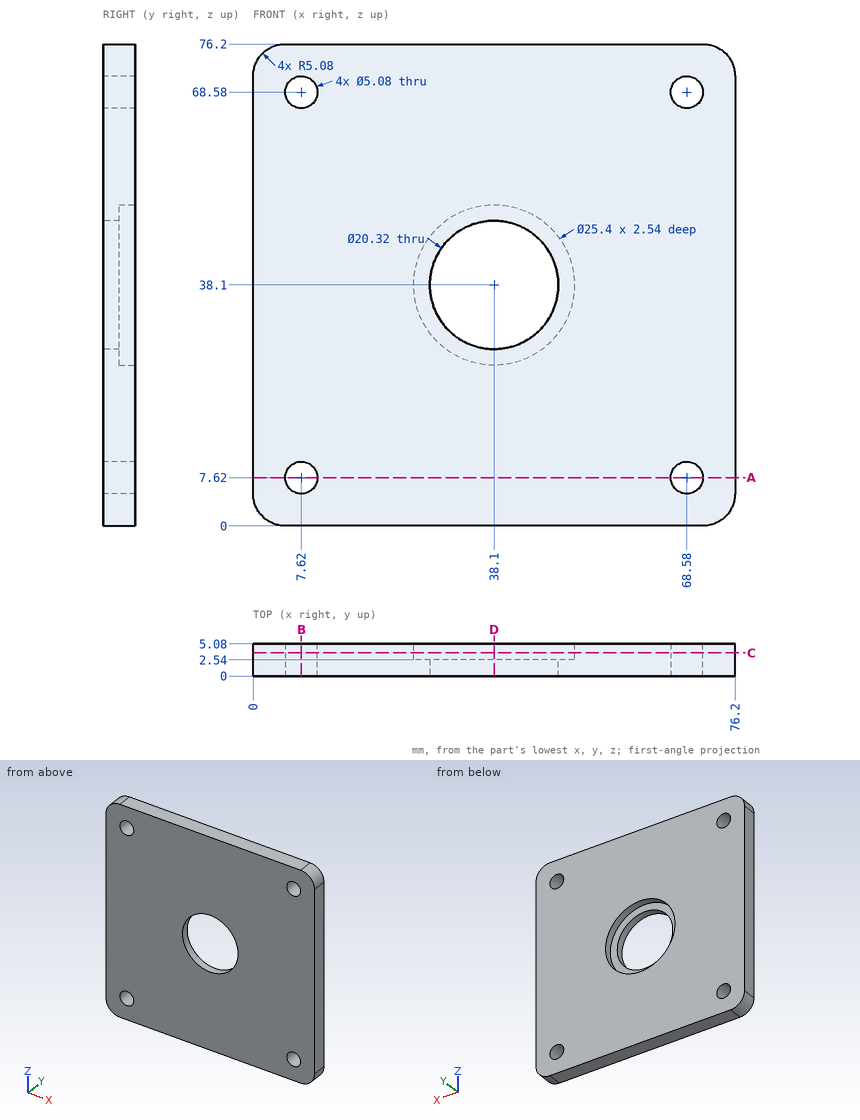
Print and shaded views of the part. All mm, measured from the part's lowest x, y and z. Round coordinates to 2 decimals unless told otherwise and drop trailing zeros. Write each loop counter-clockwise with the first axis right and the second up, starting at its lowest first coordinate (ties: lowest second). Pieces come first, ordered by that corner, then holes. Notation, with made-up numbers: (71, 61.5) - (97, 61.5) arc R21 cw to (97, 84.5) - close; hole circle Ø1 at (55.25, 12.5). An arc over 180 degrees is marked (long way). Use CSV: the item, a comma, the result in double quotes. Start each with the question number.
Item 1: Band-saw the part on B-B (x = 7.62). Write the cut outline in (y, z).
Item 2: Pin check, flat tips, straight feed: P1, Ø23, axis at x = 38.1, z = 38.1, coming from the +Y side; P2, Ø5, axis at x = 46.5, z = 47, coming from the +Y side; P3, Ø3, axis at x = 68.58, z = 68.58, coming from the -Y side. Stop position of each tip, or through.
Item 3: Band-saw the part on A-A (z = 7.62). Write the cut outline in (x, y), and give its area (3 significant figures).
Item 4: Band-saw the part on C-C (y = 3.65). Write the cut outline in (x, z).
Item 5: Band-saw the part on D-D (x = 38.1). Write the cut outline in (y, z), and give its area (3 significant figures).
Item 6: Drill centre lines: L1, parallel to Z at x = 7.62, y = 1.55; L2, parallel to X at y = 1.75, z = 67. Where is each one in solid material? Low to high. Write a range as [from, to].
Checked values:
1,outline,"(0, 0) - (5.08, 0) - (5.08, 5.08) - (0, 5.08) - close; (0, 10.16) - (5.08, 10.16) - (5.08, 66.04) - (0, 66.04) - close; (0, 71.12) - (5.08, 71.12) - (5.08, 76.2) - (0, 76.2) - close"
2,P1,"stops at y = 2.54"
2,P2,"stops at y = 5.08"
2,P3,"passes through"
3,outline,"(0, 0) - (5.08, 0) - (5.08, 5.08) - (0, 5.08) - close; (10.16, 0) - (66.04, 0) - (66.04, 5.08) - (10.16, 5.08) - close; (71.12, 0) - (76.2, 0) - (76.2, 5.08) - (71.12, 5.08) - close"
3,area,"335 mm²"
4,outline,"(0, 5.08) arc R5.08 ccw to (5.08, 0) - (71.12, 0) arc R5.08 ccw to (76.2, 5.08) - (76.2, 71.12) arc R5.08 ccw to (71.12, 76.2) - (5.08, 76.2) arc R5.08 ccw to (0, 71.12) - close; hole circle Ø5.08 at (7.62, 7.62); hole circle Ø5.08 at (7.62, 68.58); hole circle Ø25.4 at (38.1, 38.1); hole circle Ø5.08 at (68.58, 7.62); hole circle Ø5.08 at (68.58, 68.58)"
5,outline,"(0, 0) - (5.08, 0) - (5.08, 25.4) - (2.54, 25.4) - (2.54, 27.94) - (0, 27.94) - close; (0, 48.26) - (2.54, 48.26) - (2.54, 50.8) - (5.08, 50.8) - (5.08, 76.2) - (0, 76.2) - close"
5,area,"271 mm²"
6,L1,"z = [0, 5.08], [10.16, 66.04], [71.12, 76.2]"
6,L2,"x = [0, 5.63], [9.61, 66.59], [70.57, 76.2]"
